Verification items for the finished model (mm, model axes). A direction names the side the tool comes from. Give positions to 0.01 mm unless a question says otherwise; leave off trailing zeros. Write each loop counter-clockwise with the first axis right and the second up, starting at its lowest first coordinate (ties: lowest second). Pieces come first, ordered by that corner, then holes.
from build123d import *

# Parameters (mm, degrees)
F0_W     = 7.7724
F0_H     = 7.7724
F1_DEPTH = 9.6012
F2_R     = 2.4511
F3_DEPTH = 1.8796
F4_W     = 4.9784
F4_H     = 4.9784
F5_DEPTH = 8.382


with BuildPart() as f1:
    # F0 (on Top) → F1 (new body)
    with BuildSketch(Plane.XY):
        Rectangle(F0_W, F0_H)
    extrude(amount=F1_DEPTH)

    # F2 (on face) → F3 (join)
    with BuildSketch(Plane.XY.offset(9.6012)):
        Circle(F2_R)
    extrude(amount=F3_DEPTH)

    # F4 (on face) → F5 (cut)
    with BuildSketch(Plane(origin=(0, 0, 0), x_dir=(1, 0, 0), z_dir=(0, 0, -1))):
        Rectangle(F4_W, F4_H)
    extrude(amount=-F5_DEPTH, mode=Mode.SUBTRACT)


solid = f1.part
Item 1: Scan lines: line 1 along Y through (x, z) = (0, 7.25); line 2 along Z through (x, y) = (-1.75, 0.5). Record each from-to range of solid material in increasing order.
Answer key:
line 1: y = -3.89 to -2.49, 2.49 to 3.89
line 2: z = 8.38 to 11.48
Item 2: Set-up check for faces 4 (the face through (2.489, 0, 4)), 5 (the face through (0, -3.886, 5)): record each of +Z, -Z, +X, -X, +Y, -Y from which the full face is reachable in a straight line by a thin tool's end or side.
Answer key:
face 4: -Z
face 5: +Z, -Z, +X, -X, -Y
Item 3: Sectioned sample at B-B on y = 0. Record the cut outline in (x, z).
Answer key:
outline: (-3.89, 0) - (-2.49, 0) - (-2.49, 8.38) - (2.49, 8.38) - (2.49, 0) - (3.89, 0) - (3.89, 9.6) - (2.45, 9.6) - (2.45, 11.48) - (-2.45, 11.48) - (-2.45, 9.6) - (-3.89, 9.6) - close
Item 4: Sectioned sample at C-C on x = 1. Record the cut outline in (y, z), then the cut area to 3 significant figures.
Answer key:
outline: (-3.89, 0) - (-2.49, 0) - (-2.49, 8.38) - (2.49, 8.38) - (2.49, 0) - (3.89, 0) - (3.89, 9.6) - (2.24, 9.6) - (2.24, 11.48) - (-2.24, 11.48) - (-2.24, 9.6) - (-3.89, 9.6) - close
area: 41.3 mm2
Item 5: Sectioned sample at D-D on x = 2.75. Record the cut outline in (y, z), then the cut area to 3 significant figures.
Answer key:
outline: (-3.89, 0) - (3.89, 0) - (3.89, 9.6) - (-3.89, 9.6) - close
area: 74.6 mm2
Item 6: Depth check by flat-ended pin: pin 1 (2.5 mm diameter, centred on x = 1, y = -1, fed in from -Z). Enter the tip coordinate at first touch or a pass-through.
Answer key:
pin 1: stops at z = 8.38
Item 7: Release check for a two-part mould opening along Y. For faces 1 (the face through (2.338, 0.736, 10.528)), 2 (the face through (-2.489, 0, 4)), 3 (the face through (-2, 2, 9.601)) record: released by +Y, released by -Y, zero draft, split by the parting line, or undercut.
Answer key:
face 1: split by the parting line
face 2: undercut
face 3: zero draft
Item 8: Sectioned sample at A-A on z = 1.5. Record the cut outline in (x, y).
Answer key:
outline: (-3.89, -3.89) - (3.89, -3.89) - (3.89, 3.89) - (-3.89, 3.89) - close; hole (-2.49, -2.49) - (2.49, -2.49) - (2.49, 2.49) - (-2.49, 2.49) - close
